```python
from build123d import *

# Parameters (mm, degrees)
SKETCH1_R           = 55
BOSS_EXTRUDE1_DEPTH = 4
SKETCH6_W           = 87
SKETCH6_H           = 16
BOSS_EXTRUDE2_DEPTH = 4
SKETCH2_R           = 46.5
CUT_EXTRUDE1_DEPTH  = 5
SKETCH3_R           = 2.25
CUT_EXTRUDE2_DEPTH  = 5
CIRPATTERN1_COUNT   = 12
CUT_EXTRUDE3_DEPTH  = 5
SKETCH7_R           = 1.75
CUT_EXTRUDE4_DEPTH  = 5
FILLET1_R           = 4
CUT_EXTRUDE5_DEPTH  = 5


with BuildPart() as part:
    # Sketch1 → Boss-Extrude1 (new body)
    with BuildSketch(Plane(origin=(0, 0, 0), x_dir=(1, 0, 0), z_dir=(0, 1, 0))):
        Circle(SKETCH1_R)
    extrude(amount=BOSS_EXTRUDE1_DEPTH)

    # Sketch6 → Boss-Extrude2 (add)
    with BuildSketch(Plane(origin=(0, 0, 0), x_dir=(1, 0, 0), z_dir=(0, 1, 0))):
        with Locations((-43.5, 8)):
            Rectangle(SKETCH6_W, SKETCH6_H)
    extrude(amount=BOSS_EXTRUDE2_DEPTH)

    # Sketch2 → Cut-Extrude1 (cut, through all)
    with BuildSketch(Plane(origin=(0, 0, 0), x_dir=(1, 0, 0), z_dir=(0, 1, 0))):
        Circle(SKETCH2_R)
    extrude(amount=CUT_EXTRUDE1_DEPTH, mode=Mode.SUBTRACT)

    # Sketch3 → Cut-Extrude2 (cut, through all)
    with BuildSketch(Plane(origin=(0, 0, 0), x_dir=(1, 0, 0), z_dir=(0, 1, 0))):
        with Locations((-50.805929603, 4.44494288)):
            Circle(SKETCH3_R)
    cut_extrude2 = extrude(amount=CUT_EXTRUDE2_DEPTH, mode=Mode.SUBTRACT)

    # CirPattern1: Cut-Extrude2 ×12 about axis
    cirpattern1_axis = Axis((0, 0, 0), (0, 1, 0))
    for i in range(1, CIRPATTERN1_COUNT):
        add(cut_extrude2.rotate(cirpattern1_axis, i * 360 / CIRPATTERN1_COUNT), mode=Mode.SUBTRACT)

    # Sketch4 → Cut-Extrude3 (cut, through all)
    with BuildSketch(Plane(origin=(0, 0, 0), x_dir=(1, 0, 0), z_dir=(0, 1, 0))):
        with BuildLine():
            Line((0, 0), (-62.402274146, 0))
            ThreePointArc((-62.402274146, 0), (58.638956535, -21.342834747), (-47.802915347, 40.111408637))
            Line((-47.802915347, 40.111408637), (0, 0))
        make_face()
    extrude(amount=CUT_EXTRUDE3_DEPTH, mode=Mode.SUBTRACT)

    # Sketch7 → Cut-Extrude4 (cut, through all)
    with BuildSketch(Plane(origin=(0, 0, 0), x_dir=(1, 0, 0), z_dir=(0, 1, 0))):
        with Locations((-61.8, 12.6)):
            Circle(SKETCH7_R)
        with Locations((-84, 2.3)):
            Circle(SKETCH7_R)
    extrude(amount=CUT_EXTRUDE4_DEPTH, mode=Mode.SUBTRACT)

    # Fillet1
    fillet1_edges = [part.edges().sort_by_distance(p)[0] for p in [
        (-46.5, 2, 0),
    ]]
    fillet(fillet1_edges, radius=FILLET1_R)

    # Sketch8 → Cut-Extrude5 (cut, through all)
    with BuildSketch(Plane(origin=(0, 0, 0), x_dir=(1, 0, 0), z_dir=(0, 1, 0))):
        with BuildLine():
            Line((-39.970362944, 27.909363771), (-43.650121746, 30.47876068))
            ThreePointArc((-43.650121746, 30.47876068), (-50.07963309, 18.064283285), (-53.055558124, 4.404058716))
            Line((-53.055558124, 4.404058716), (-48.582909499, 4.032791164))
            ThreePointArc((-48.582909499, 4.032791164), (-45.857858596, 16.541442048), (-39.970362944, 27.909363771))
        make_face()
    extrude(amount=CUT_EXTRUDE5_DEPTH, mode=Mode.SUBTRACT)


solid = part.part
```
Geometry: final body of the model. Coordinates: model frame, mm. A direction names the side the tool comes from. Coordinates: 2 decimals unless noted, no trailing zeros. Write each loop counter-clockwise with the first axis right and the second up, starting at its lowest first coordinate (ties: lowest second). Pieces come first, ordered by that corner, then holes. Notation, with made-up numbers: M 24.25,-19 L 36.25,-19 A22 cw 36.25,19 Z; hole C -9,66.5 d5. An arc over 180 degrees is marked long. Answer as CSV lines item,"result". Start each with the question number.
Q1. Pin query (flat end, axial travel): P1, Ø2, axis at x = -68.5, y = 2.5, coming from the -Z side. Return the tip coordinate at first contact, or that it passes through.
Q2. Line query: line 1 (Z direction, x = -61.8, y = 1.7); line 2 (Z direction, x = -84, y = 2.2); line 3 (X direction, y = 3.65, z = -11). Output: solid intervals per line, ascending. Write a range as from..to.
Q3. Cut plane A-A on x = -84. Return the cut outline in (y, z).
Q4. Cut plane C-C on y = 0.5. Count the separate pieces of the cut face and the enclosed holes in it, then the cut area to 3 significant figures.
Q5. Cut plane B-B on z = -12.6. Return the cut outline in (x, y), then the cut area to 3 significant figures.
Q6. Mould query, pull axis X, two halves, no side actions, for faces 1 (the cylindrical face through (-48.281, 1.972, -26.343)), 2 (the cylindrical face through (-45.92, 1.97, -16.37)), 3 (the cylindrical face through (-63.55, 1.97, -12.68)), 4 (the flat face through (-70, 2, -16)). Classes: released by +X, released by -X, zero draft, split by the parting line, or undercut.
Q7. Cut plane D-D on z = -8. Return the cut outline in (x, y).
Q8. Reachability of faces 5 (the flat face through (-87, 2, -8)), 6 (the cylindrical face through (-49.96, 1.97, -18.39)) from +Z, -Z, +X, -X, +Y, -Y: full face, straight path, thin tool, end or side. Return the list, or none.
Findings below:
1,P1,"stops at z = -16"
2,line 1,"z = -16..-14.35, -10.85..0"
2,line 2,"z = -16..-4.05, -0.55..0"
2,line 3,"x = -87..-62.51, -61.09..-52.09, -47.49..-45.18"
3,outline,"M 0,-16 L 4,-16 L 4,-4.05 L 0,-4.05 Z; M 0,-0.55 L 4,-0.55 L 4,0 L 0,0 Z"
4,separate pieces,"1"
4,enclosed holes,"3"
4,area,"668 mm2"
5,outline,"M -87,0 L -63.55,0 L -63.55,4 L -87,4 Z; M -60.05,0 L -51.73,0 L -51.73,4 L -60.05,4 Z; M -47.09,0 L -44.76,0 L -44.76,4 L -47.09,4 Z"
5,area,"136 mm2"
6,face 1,"released by -X"
6,face 2,"undercut"
6,face 3,"undercut"
6,face 4,"zero draft"
7,outline,"M -87,0 L -52.63,0 L -52.63,4 L -87,4 Z; M -48.09,0 L -45.81,0 L -45.81,4 L -48.09,4 Z"
8,face 5,"+Z, -Z, -X, +Y, -Y"
8,face 6,"+Y, -Y"
